Work out the finished part from the listing and answer in its coordinate system (mm). Face numbers are marked on the shaded views. Round coordinates to 2 decimals unless told otherwise and drop trailing zeros. Loops run counter-clockwise (first coordinate to the right, second up) from the corner with the lowest first, then second, coordinate; pieces in that order, holes last. Notation, with made-up numbers: (-31.5, 86.5) - (22.5, 86.5) arc R15 cw to (22.5, 100.5) - close; hole circle Ø10 at (-15.75, 21). An arc over 180 degrees is marked (long way). Return JSON: item names as keys, results as strings.
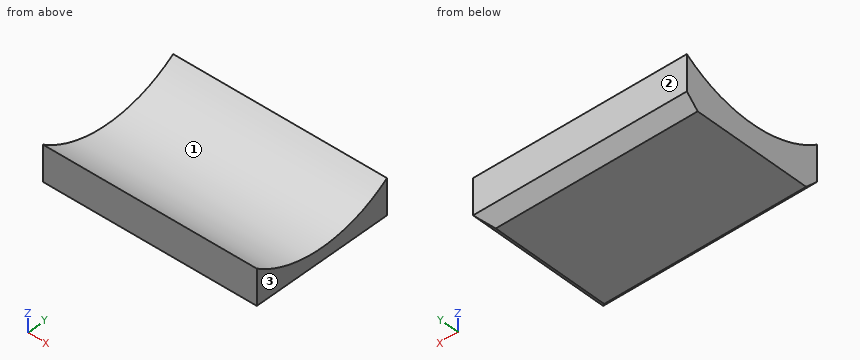
from build123d import *

# Parameters (mm, degrees)
F0_W     = 457.2
F0_H     = 304.8
F1_DEPTH = 50.8
F2_R     = 258.858345
F3_DEPTH = 457.2
F4_SIZE  = 25.4
F5_SIZE  = 25.4


with BuildPart() as f1:
    # F0 (on Top) → F1 (new body, symmetric)
    with BuildSketch(Plane.XY):
        Rectangle(F0_W, F0_H)
    extrude(amount=F1_DEPTH, both=True)

    # F2 (on face) → F3 (cut, through all)
    with BuildSketch(Plane.YZ.offset(228.6)):
        with Locations((0, 260.041207)):
            Circle(F2_R)
    extrude(amount=-F3_DEPTH, mode=Mode.SUBTRACT)

    # F4
    f4_edges = [f1.edges().sort_by_distance(p)[0] for p in [
        (0, -152.4, -50.8),
    ]]
    chamfer(f4_edges, length=F4_SIZE)

    # F5
    f5_edges = [f1.edges().sort_by_distance(p)[0] for p in [
        (228.6, 12.7, -50.8),
        (0, 152.4, -50.8),
    ]]
    chamfer(f5_edges, length=F5_SIZE)


solid = f1.part
1) Section D-D (z = 7) is taken. Give the vertices of the cut face in (x, y).
Verdict:
{"outline": "(-228.6, -152.4) - (228.6, -152.4) - (228.6, -54.57) - (-228.6, -54.57) - close; (-228.6, 54.57) - (228.6, 54.57) - (228.6, 152.4) - (-228.6, 152.4) - close"}
2) Section A-A (z = 37) is taken. Give the vertices of the cut face in (x, y).
Verdict:
{"outline": "(-228.6, -152.4) - (228.6, -152.4) - (228.6, -131.38) - (-228.6, -131.38) - close; (-228.6, 131.38) - (228.6, 131.38) - (228.6, 152.4) - (-228.6, 152.4) - close"}
3) Find the intervals of material crossed by L1, parallel to Y at x = 76, z = 34; L2, parallel to Y at x = -135.5, z = 29; L3, parallel to X at y = -83.5, z = -25.5, in increasing order.
Verdict:
{"L1": "y = -152.4 to -126.15, 126.15 to 152.4", "L2": "y = -152.4 to -116.74, 116.74 to 152.4", "L3": "x = -228.6 to 228.5"}
4) Section B-B (x = -198.5) is taken. Give the vertices of the cut face in (y, z), and give its area (3 significant figures).
Verdict:
{"outline": "(-152.4, -25.4) - (-127, -50.8) - (127, -50.8) - (152.4, -25.4) - (152.4, 50.8) arc R258.86 cw to (-152.4, 50.8) - close", "area": "20,000 mm2"}
5) Determine the mould class of the marked faces 1, 2 and 3 for opening direction Y: pulls with the +Y half, pulls with the -Y half, needs draft (parallel to the pull), parting line crosses it, or undercut.
Verdict:
{"face 1": "undercut", "face 2": "pulls with the +Y half", "face 3": "needs draft"}
6) Section C-C (y = -68) is taken. Give the vertices of the cut face in (x, z).
Verdict:
{"outline": "(-228.6, -50.8) - (203.2, -50.8) - (228.6, -25.4) - (228.6, 10.27) - (-228.6, 10.27) - close"}
